The figure shows three views and two pictorial views of one solid part (mm, origin at its lowest corner). Answer the questions. A direction names the side the tool comes from. Give positions to 0.01 mm unless a question says otherwise; leave off trailing zeros. Write each loop counter-clockwise with the first axis right and the second up, starting at its lowest first coordinate (ties: lowest second). Pieces come first, ordered by that corner, then holes. Notation, with made-up numbers: M 87.25,60.25 L 123.25,60.25 A6 ccw 123.25,70.25 Z; hole C 31.5,63.5 d3. An arc over 180 degrees is marked long. Answer as CSV lines item,"result". Start each with the question number.
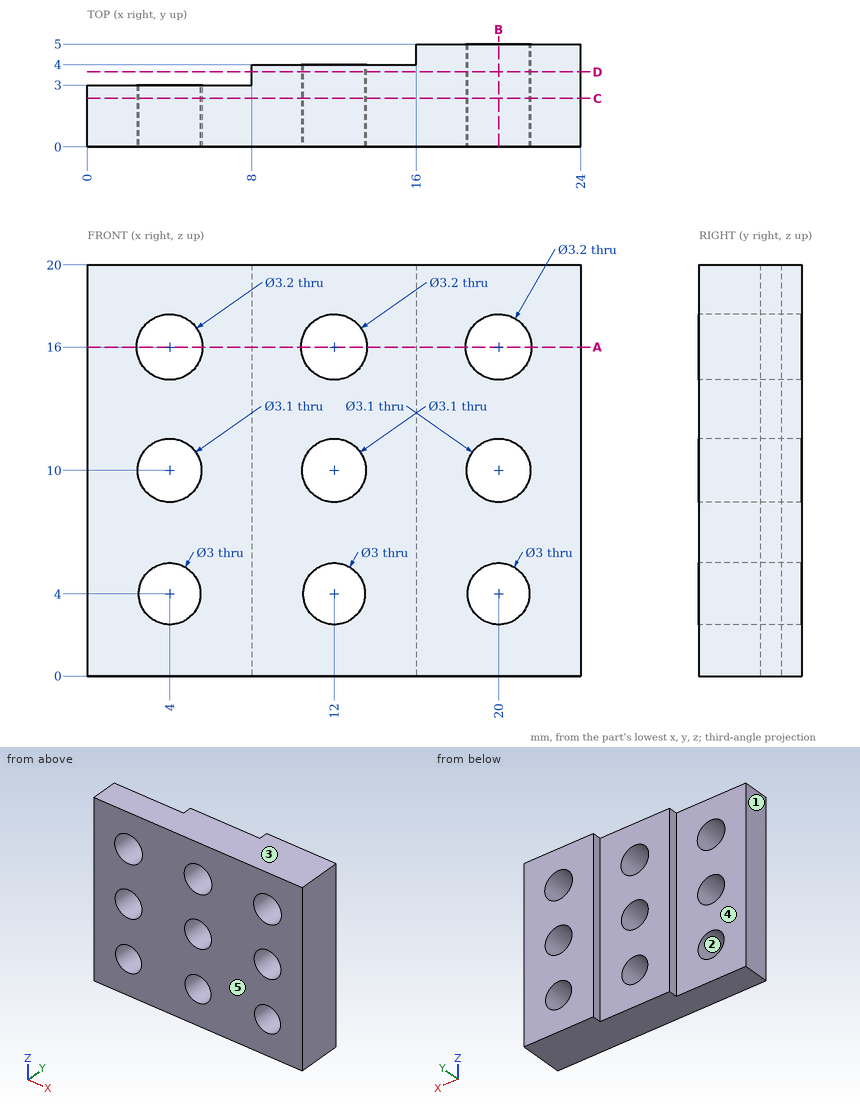
1. Find section D-D on y = 3.65. Determine the outline of the cut face in (x, z).
2. Find section A-A on z = 16. Determine the outline of the cut face in (x, y), then the cut area to 3 significant figures.
3. Given pin 1 (1 mm diameter, centred on y = 4, z = 6.5, fed in from -X); pin 2 (12 mm diameter, centred on x = 3.5, z = 6, fed in from -Y); pin 3 (9 mm diameter, centred on x = 10, z = 13, fed in from +Y); pin 4 (1.8 mm diameter, centred on x = 20, z = 4, fed in from -Y), each flat-ended and moving along its own axis, determine where each tip first touches the part or whether it passes through.
4. Find the intervals of material crossed by line 1 (Z direction, x = 12, y = 1.45); line 2 (X direction, y = 1.6, z = 4); line 3 (X direction, y = 1.7, z = 15), in increasing order. Write a range as [from, to].
5. For the marked faces 4 and 5, determine the directions among +Z, -Z, +X, -X, +Y, -Y from which every point of the face is accessible in a straight line to the end or side of a thin tool.
6. Determine the mould class of the marked faces 1, 2 and 3 for opening direction Z: +Z half, -Z half, draft (parallel to the pull), parting line (faces both ways), or undercut.
7. Find section B-B on x = 20. Determine the outline of the cut face in (y, z), then the cut area to 3 significant figures.
8. Find section C-C on y = 2.35. State how many separate pieces and enclosed holes the cut face has, then the cut area to 3 significant figures.
Computed:
1,outline,"M 8,0 L 24,0 L 24,20 L 8,20 Z; hole C 12,16 d3.2; hole C 12,10 d3.1; hole C 12,4 d3; hole C 20,16 d3.2; hole C 20,10 d3.1; hole C 20,4 d3"
2,outline,"M 0,0 L 2.4,0 L 2.4,3 L 0,3 Z; M 5.6,0 L 10.4,0 L 10.4,4 L 8,4 L 8,3 L 5.6,3 Z; M 13.6,0 L 18.4,0 L 18.4,5 L 16,5 L 16,4 L 13.6,4 Z; M 21.6,0 L 24,0 L 24,5 L 21.6,5 Z"
2,area,"57.6 mm^2"
3,pin 1,"stops at x = 8"
3,pin 2,"stops at y = 0"
3,pin 3,"stops at y = 4"
3,pin 4,"passes through"
4,line 1,"z = [0, 2.5], [5.5, 8.45], [11.55, 14.4], [17.6, 20]"
4,line 2,"x = [0, 2.5], [5.5, 10.5], [13.5, 18.5], [21.5, 24]"
4,line 3,"x = [0, 2.75], [5.25, 10.75], [13.25, 18.75], [21.25, 24]"
5,face 4,"+Z, -Z, -X, +Y"
5,face 5,"+Z, -Z, +X, -X, -Y"
6,face 1,"draft"
6,face 2,"undercut"
6,face 3,"+Z half"
7,outline,"M 0,0 L 5,0 L 5,2.5 L 0,2.5 Z; M 0,5.5 L 5,5.5 L 5,8.45 L 0,8.45 Z; M 0,11.55 L 5,11.55 L 5,14.4 L 0,14.4 Z; M 0,17.6 L 5,17.6 L 5,20 L 0,20 Z"
7,area,"53.5 mm^2"
8,separate pieces,"1"
8,enclosed holes,"9"
8,area,"412 mm^2"
